Autodesk Inventor part; units mm, degrees
ref_plane "YZ Plane" through (0, 0, 0) normal (1, 0, 0) x (0, 1, 0)
ref_plane "XZ Plane" through (0, 0, 0) normal (0, 1, 0) x (-1, 0, 0)
ref_plane "XY Plane" through (0, 0, 0) normal (0, 0, 1) x (1, 0, 0)
sketch "Sketch1" plane through (0, 0, 0) normal (0, 1, 0) x (-1, 0, 0)
  line L0 (0, 0) -> (-25.4, 0)
  line L1 (-25.4, 0) -> (-25.4, -3.175)
  line L2 (-25.4, -3.175) -> (0, -3.175)
  line L3 (0, -3.175) -> (0, 0)
  line L4 (-25.4, 0) -> (-22.225, 0)
  line L5 (-22.225, 0) -> (-22.225, -25.4)
  line L6 (-22.225, -25.4) -> (-25.4, -25.4)
  line L7 (-25.4, -25.4) -> (-25.4, 0)
  dimension "d0" = 25.4
  dimension "d1" = 3.175
  dimension "d2" = 25.4
  dimension "d3" = 3.175
extrude "Extrusion1" add sketch "Sketch1" along normal blind 76.2
sketch "Sketch2" plane through (25.4, 0, 0) normal (1, 0, 0) x (0, 0, -1)
  line L0 (0, 0) -> (0, 76.2)
  line L1 (0, 76.2) -> (12.7, 76.2)
  line L2 (12.7, 76.2) -> (12.7, 57.15)
  line L3 (0, 0) -> (25.4, 0)
  line L4 (12.7, 0) -> (12.7, 19.05)
  circle A0 centre (12.7, 57.15) radius 2.54
  circle A1 centre (12.7, 19.05) radius 2.54
  dimension "d6" = 12.7
  dimension "d7" = 19.05
  dimension "d8" = 19.05
  dimension "d9" = 5.08
extrude "Extrusion2" cut sketch "Sketch2" against normal blind 25.4
sketch "Sketch3" plane through (0, 0, 0) normal (0, 0, 1) x (1, 0, 0)
  line L0 (0, 0) -> (0, 76.2)
  line L1 (0, 76.2) -> (12.7, 76.2)
  line L2 (0, 76.2) -> (25.4, 76.2)
  line L3 (12.7, 76.2) -> (12.7, 57.15)
  line L4 (12.7, 0) -> (12.7, 19.05)
  circle A0 centre (12.7, 57.15) radius 2.54
  circle A1 centre (12.7, 19.05) radius 2.54
  dimension "d12" = 19.05
  dimension "d13" = 19.05
  dimension "d14" = 5.08
extrude "Extrusion3" cut sketch "Sketch3" against normal blind 25.4
properties part number "L Bracket 3in" material "Aluminum 6061"
The model under review builds one solid part; all positions refer to its coordinate system, in mm. A direction names the side the tool comes from. Round coordinates to 2 decimals unless told otherwise and drop trailing zeros. Write each loop counter-clockwise with the first axis right and the second up, starting at its lowest first coordinate (ties: lowest second). Pieces come first, ordered by that corner, then holes. Notation, with made-up numbers: (63.5, 48) - (113.5, 48) arc R15 cw to (113.5, 70) - close; hole circle Ø10 at (40, -11). An arc over 180 degrees is marked (long way). One line per question, with ' | ' between items.
Item 1: For P1, Ø4, axis at x = 12.7, y = 57.15, coming from the -Z side; P2, Ø12, axis at x = 10.5, y = 24, coming from the -Z side (3 decimals), all flat-tipped, find the tip position at first contact; note any pin that passes through.
Resolved:
P1: passes through | P2: stops at z = -3.175
Item 2: The part is to be moulded in two halves that separate along X. For faces 1 (the face through (12.15, 54.67, -1.57)), 2 (the face through (0, 38, -2)), 3 (the face through (25.4, 38, -13)), 4 (the face through (24, 38, -25.4)), say which applies: pulls with the +X half, pulls with the -X half, needs draft (parallel to the pull), parting line crosses it, or undercut.
Resolved:
face 1: undercut | face 2: pulls with the -X half | face 3: pulls with the +X half | face 4: needs draft
Item 3: For faces 5 (the face through (11, 38, -3.175)), 6 (the face through (23.83, 16.57, -12.15)), list the 3-axis set-ups (+Z, -Z, +X, -X, +Y, -Y) from which the entire face can be reached by the end or side of a thin tool; tool diameter is ignored.
Resolved:
face 5: -Z, -X, +Y, -Y | face 6: +X, -X
Item 4: Add section B-B, the plane z = -12.7. Give the boundary of the cut face in (x, y) (3 decimals), then the cut area to 3 significant figures.
Resolved:
outline: (22.225, 0) - (25.4, 0) - (25.4, 16.51) - (22.225, 16.51) - close; (22.225, 21.59) - (25.4, 21.59) - (25.4, 54.61) - (22.225, 54.61) - close; (22.225, 59.69) - (25.4, 59.69) - (25.4, 76.2) - (22.225, 76.2) - close | area: 210 mm2
Item 5: Add section A-A, the plane y = 19.05. Give the boundary of the cut face in (x, z) (3 decimals), then the cut area to 3 significant figures.
Resolved:
outline: (0, -3.175) - (10.16, -3.175) - (10.16, 0) - (0, 0) - close; (15.24, -3.175) - (22.225, -3.175) - (22.225, -10.16) - (25.4, -10.16) - (25.4, 0) - (15.24, 0) - close; (22.225, -25.4) - (25.4, -25.4) - (25.4, -15.24) - (22.225, -15.24) - close | area: 119 mm2
Item 6: To check wall thickness, follow probe 1 along Y at (x, z) = (12.7, -1.05); probe 2 along X at (y, z) = (19.05, -2); probe 3 along Z at (x, y) = (23.1, 19.05). State the ranges of each line that lie inside material, in increasing order.
Resolved:
probe 1: y = 0 to 16.51, 21.59 to 54.61, 59.69 to 76.2 | probe 2: x = 0 to 10.16, 15.24 to 25.4 | probe 3: z = -25.4 to -15.24, -10.16 to 0
Item 7: Add section C-C, the plane x = 12.7. Give the boundary of the cut face in (y, z) (3 decimals).
Resolved:
outline: (0, -3.175) - (16.51, -3.175) - (16.51, 0) - (0, 0) - close; (21.59, -3.175) - (54.61, -3.175) - (54.61, 0) - (21.59, 0) - close; (59.69, -3.175) - (76.2, -3.175) - (76.2, 0) - (59.69, 0) - close
Item 8: Add section D-D, the plane x = 23.75. Give the boundary of the cut face in (y, z), then the cut area to 3 significant figures.
Resolved:
outline: (0, -25.4) - (76.2, -25.4) - (76.2, 0) - (0, 0) - close; hole circle Ø5.08 at (19.05, -12.7); hole circle Ø5.08 at (57.15, -12.7) | area: 1,890 mm2
